CAD build for the part. Positions are in the model's coordinates, mm. Face numbers are marked on the shaded views. A direction names the side the tool comes from. Round coordinates to 2 decimals unless told otherwise and drop trailing zeros. Put each result on its own line as item: value. Start each with the question number.
Item 1: Pin check, flat tips, straight feed: pin 1 Ø1.4 at (y, z) = (-22, 2) entering from -X; pin 2 Ø24 at (y, z) = (-31, 41.5) entering from +X; pin 3 Ø3 at (y, z) = (-39.5, 10) entering from -X. Stop position of each tip, or through.
Item 2: 3-axis set-ups, long thin cutter, end or side, ignore diameter. For the marked faces 1, 2 and 3: which of +Z, -Z, +X, -X, +Y, -Y reach the whole face in a straight line?
Item 3: Drill centre lines: line 1 (Y direction, x = 39.5, z = 17); line 2 (X direction, y = -20.5, z = 34); line 3 (Z direction, x = 21, y = -14). Where is each one in solid material? Low to high. Write a range as from..to.
Item 4: Mould opens along X. For the marked faces 4, 5, 6 and 7 say: released by +X, released by -X, zero draft, split by the parting line, or undercut.
```python
from build123d import *

# Parameters (mm, degrees)
F0_W     = 5.08
F0_H     = 4.445
F1_DEPTH = 5.08
F2_DEPTH = 55.88
F4_SIZE  = 5.07999


# Not quite as in the source:
# - a fillet or chamfer is up to 0.001 mm smaller than in the source, because OpenCascade refuses the exact size


with BuildPart() as f1:
    # F0 (on Top) → F1 (new body)
    with BuildSketch(Plane.XY):
        Polygon((0, -50.8), (0, 0), (50.8, 0), (50.8, -23.1775), (55.88, -23.1775), (55.88, 5.08), (-5.08, 5.08), (-5.08, -55.88), (55.88, -55.88), (55.88, -27.6225), (50.8, -27.6225), (50.8, -50.8), align=None)
        with Locations((53.34, -25.4)):
            Rectangle(F0_W, F0_H)
        Polygon((28.8019571453, -23.1775), (49.53, -23.1775), (49.53, -1.27), (1.27, -1.27), (1.27, -49.53), (49.53, -49.53), (49.53, -27.6225), (28.8019571453, -27.6225), (28.8019571453, -30.439995), (21.8463055789, -30.439995), (21.8463055789, -20.360005), (28.8019571453, -20.360005), align=None)
        Polygon((50.8, 0), (0, 0), (0, -50.8), (50.8, -50.8), (50.8, -27.6225), (49.53, -27.6225), (49.53, -49.53), (1.27, -49.53), (1.27, -1.27), (49.53, -1.27), (49.53, -23.1775), (50.8, -23.1775), align=None)
    extrude(amount=F1_DEPTH)

    # F0 (on Top) → F2 (join)
    with BuildSketch(Plane.XY):
        Polygon((50.8, 0), (0, 0), (0, -50.8), (50.8, -50.8), (50.8, -27.6225), (49.53, -27.6225), (49.53, -49.53), (1.27, -49.53), (1.27, -1.27), (49.53, -1.27), (49.53, -23.1775), (50.8, -23.1775), align=None)
    extrude(amount=F2_DEPTH)

    # F4 (size 5.08 in the source; OpenCascade refuses exactly that, so slightly less here)
    f4_edges = [f1.edges().sort_by_distance(p)[0] for p in [
        (-5.08, -25.4, 5.08),
        (25.4, -55.88, 5.08),
        (55.88, -25.4, 5.08),
        (25.4, 5.08, 5.08),
    ]]
    chamfer(f4_edges, length=F4_SIZE)


solid = f1.part
```
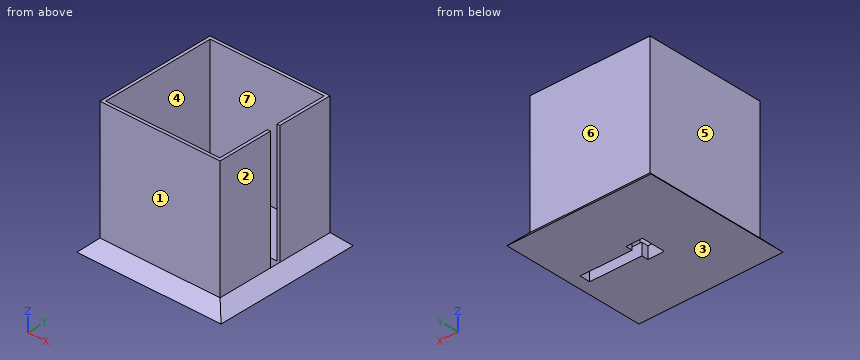
Output values:
1. pin 1: x = -3.78
1. pin 2: x = 50.8
1. pin 3: x = 0
2. face 1: +Z, +X, -X, -Y
2. face 2: +Z, +X, +Y, -Y
2. face 3: -Z, +X, -X, +Y, -Y
3. line 1: -50.8..-49.53, -1.27..0
3. line 2: 0..1.27, 49.53..50.8
3. line 3: 0..5.08
4. face 4: undercut
4. face 5: released by -X
4. face 6: zero draft
4. face 7: undercut
